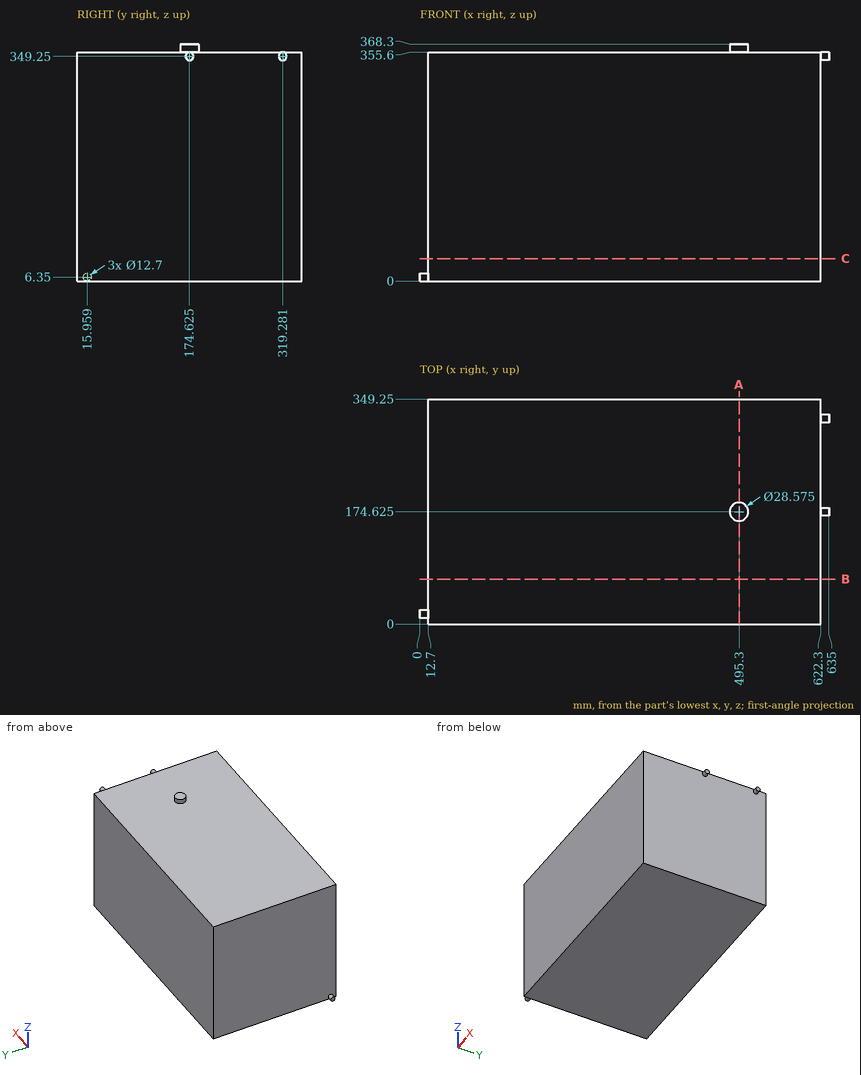
Geometry check sheet. Reference: drawing and pictorial views, mm from the part's lowest x, y, z. Coordinates: 2 decimals unless noted, no trailing zeros. Order: outer loops, then holes, each group sorted by start corner. A loop starts at its lowest first (then second) coordinate and runs counter-clockwise, first axis right, second up. Notation, with made-up numbers: (65.5, 5.5) - (113.5, 5.5) arc R25 cw to (113.5, 31.5) - close; hole circle Ø4 at (7.5, -36). An arc over 180 degrees is marked (long way). One line per item, written item: value.
(1) Thickness scan on probe 1 along Z at (x, y) = (227, 96); probe 2 along X at (y, z) = (226, 333). Record the ranges inside material, lowest first. Write a range as from..to.
Data:
probe 1: z = 0..355.6
probe 2: x = 12.7..622.3
(2) Sectioned sample at B-B (y = 70). Enter the section's corners in (x, z), and give its area (3 significant figures).
Data:
outline: (12.7, 0) - (622.3, 0) - (622.3, 355.6) - (12.7, 355.6) - close
area: 217,000 mm^2
(3) Sectioned sample at A-A (x = 495.3). Enter the section's corners in (y, z).
Data:
outline: (0, 0) - (349.25, 0) - (349.25, 355.6) - (188.91, 355.6) - (188.91, 368.3) - (160.34, 368.3) - (160.34, 355.6) - (0, 355.6) - close
(4) Depth check by flat-ended pin: pin 1 Ø3 at (x, z) = (385.5, 74.5) entering from -Y; pin 2 Ø2 at (x, y) = (533, 301.5) entering from +Z; pin 3 Ø6 at (y, z) = (101.5, 221) entering from -X; pin 4 Ø2 at (y, z) = (197, 276.5) entering from +X. Enter the tip coordinate at first touch or a pass-through.
Data:
pin 1: stops at y = 0
pin 2: stops at z = 355.6
pin 3: stops at x = 12.7
pin 4: stops at x = 622.3
(5) Sectioned sample at C-C (z = 35). Enter the section's corners in (x, y).
Data:
outline: (12.7, 0) - (622.3, 0) - (622.3, 349.25) - (12.7, 349.25) - close
